```python
from build123d import *

# Parameters (mm, degrees)
SKETCH1_R           = 5.71
BOSS_EXTRUDE1_DEPTH = 25.23


with BuildPart() as part:
    # Sketch1 → Boss-Extrude1 (new body)
    with BuildSketch(Plane.YZ):
        Polygon((0, 12.615), (-637.845, 12.615), (-207.569, -310.092), (-200, -312.615), (200, -312.615), (207.569, -310.092), (637.845, 12.615), align=None)
        with Locations(Location((-600, 0, 0), (0, 0, 270))):
            Circle(SKETCH1_R, mode=Mode.SUBTRACT)
        with Locations(Location((0, 0, 0), (0, 0, 270))):
            Circle(SKETCH1_R, mode=Mode.SUBTRACT)
        with Locations(Location((-200, -300, 0), (0, 0, 270))):
            Circle(SKETCH1_R, mode=Mode.SUBTRACT)
        with Locations(Location((200, -300, 0), (0, 0, 270))):
            Circle(SKETCH1_R, mode=Mode.SUBTRACT)
        with Locations(Location((600, 0, 0), (0, 0, 270))):
            Circle(SKETCH1_R, mode=Mode.SUBTRACT)
        Polygon((176.428656887, -287.385), (0, -22.74201467), (-176.428656887, -287.385), align=None, mode=Mode.SUBTRACT)
        Polygon((-562.155, -12.615), (-203.099228742, -281.906828443), (-23.571343113, -12.615), align=None, mode=Mode.SUBTRACT)
        Polygon((203.099228742, -281.906828443), (562.155, -12.615), (23.571343113, -12.615), align=None, mode=Mode.SUBTRACT)
    extrude(amount=BOSS_EXTRUDE1_DEPTH)


solid = part.part
```
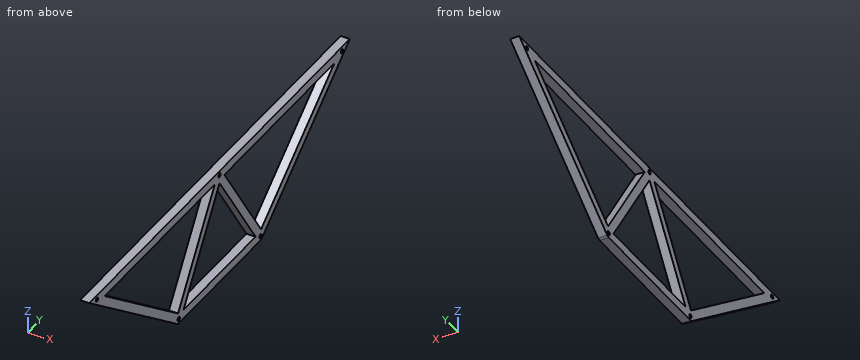
The listing builds one solid part. Answer for the finished solid, in the listing's coordinates (mm). Round coordinates to 2 decimals unless told otherwise and drop trailing zeros. Loops run counter-clockwise (first coordinate to the right, second up) from the corner with the lowest first, then second, coordinate; pieces in that order, holes last. Notation, with made-up numbers: (-38, 14) - (13, 14) arc R24 ccw to (13, 33) - close; hole circle Ø10 at (82.5, -27). An arc over 180 degrees is marked (long way). Return JSON: item names as keys, results as strings. Group by question number.
1. The part is cut by section B-B on y = -39. Determine the outline of the cut face in (x, z) (3 decimals).
2. The part is cut by section A-A on x = 5.5. State how many separate pieces and enclosed holes the cut face has, then the cut area to 3 significant figures.
3. Each of these flat-tipped pins is pushed along its axis until it touches: P1, Ø18.5, axis at y = -200, z = -300, coming from the -X side; P2, Ø3, axis at x = 12.5, z = -202, coming from the -Y side; P3, Ø6, axis at x = 4.5, z = -181.5, coming from the +Y side (3 decimals); P4, Ø6, axis at x = 10.5, z = -77.5, coming from the +Y side. Where does it stop, or does it pass through?
4. Consider probe 1 along Y at (x, z) = (10.75, -300) (3 decimals); probe 2 along Y at (x, z) = (16.25, 0) (3 decimals); probe 3 along Y at (x, z) = (3.5, -111) (3 decimals). Determine where each line is inside the solid, lowest interval first.
5. The part is cut by section C-C on z = -220. Determine the outline of the cut face in (x, y), then the cut area to 3 significant figures.
6. The part is cut by section D-D on y = 347.5. Determine the outline of the cut face in (x, z) (3 decimals), then the cut area to 3 significant figures.
Resolved:
{
 "1": {"outline": "(0, -312.615) - (25.23, -312.615) - (25.23, -287.385) - (0, -287.385) - close; (0, -81.242) - (25.23, -81.242) - (25.23, -35.758) - (0, -35.758) - close; (0, -12.615) - (25.23, -12.615) - (25.23, 12.615) - (0, 12.615) - close"},
 "2": {"separate pieces": "1", "enclosed holes": "8", "area": "81,600 mm²"},
 "3": {"P1": "stops at x = 0", "P2": "stops at y = -353.69", "P3": "stops at y = 383.025", "P4": "stops at y = 521.69"},
 "4": {"probe 1": "y = -221.025 to -205.71, -194.29 to 194.29, 205.71 to 221.025", "probe 2": "y = -621.025 to -605.71, -594.29 to -5.71, 5.71 to 594.29, 605.71 to 621.025", "probe 3": "y = -473.025 to -430.975, -89.161 to -58.839, 58.839 to 89.161, 430.975 to 473.025"},
 "5": {"outline": "(0, -327.69) - (25.23, -327.69) - (25.23, -285.64) - (0, -285.64) - close; (0, -161.83) - (25.23, -161.83) - (25.23, -131.51) - (0, -131.51) - close; (0, 131.51) - (25.23, 131.51) - (25.23, 161.83) - (0, 161.83) - close; (0, 285.64) - (25.23, 285.64) - (25.23, 327.69) - (0, 327.69) - close", "area": "3,650 mm²"},
 "6": {"outline": "(0, -205.144) - (25.23, -205.144) - (25.23, -173.606) - (0, -173.606) - close; (0, -12.615) - (25.23, -12.615) - (25.23, 12.615) - (0, 12.615) - close", "area": "1,430 mm²"}
}
